```python
from build123d import *
from OCP.BRepFilletAPI import BRepFilletAPI_MakeChamfer

# Parameters (mm, degrees)
SKETCH1_R           = 0.85
BOSS_EXTRUDE1_DEPTH = 5
BOSS_EXTRUDE2_DEPTH = 2
SKETCH3_R           = 2.25
BOSS_EXTRUDE3_DEPTH = 5
SKETCH4_R           = 3.5
CUT_EXTRUDE1_DEPTH  = 3
SKETCH5_W           = 10
SKETCH5_H           = 10
CUT_EXTRUDE2_DEPTH  = 47.770717335
FILLET1_R           = 7
CHAMFER3_SIZE       = 0.5
CHAMFER1_SIZE       = 2.5
CHAMFER1_SIZE_2     = 1.25


with BuildPart() as part:
    # Sketch1 → Boss-Extrude1 (new body)
    with BuildSketch(Plane.XY):
        Polygon((-11, -35), (-11, 29), (10, 29), (10, -35), (17.5, -35), (17.5, 37.5), (-17.5, 37.5), (-17.5, -35), align=None)
        with Locations((-12.5, 32.5)):
            Circle(SKETCH1_R, mode=Mode.SUBTRACT)
        with Locations((12.5, 32.5)):
            Circle(SKETCH1_R, mode=Mode.SUBTRACT)
        with Locations((12.5, -32.5)):
            Circle(SKETCH1_R, mode=Mode.SUBTRACT)
    extrude(amount=BOSS_EXTRUDE1_DEPTH)

    # Sketch2 → Boss-Extrude2 (add)
    with BuildSketch(Plane.XY):
        Polygon((17.5, -35), (17.5, 37.5), (-17.5, 37.5), (-17.5, -35), (-15.1, -35), (-15.1, 35.1), (15.1, 35.1), (15.1, -35), align=None)
    extrude(amount=-BOSS_EXTRUDE2_DEPTH)

    # Sketch3 → Boss-Extrude3 (add)
    # profile 1 of 2: a face of its own
    with BuildSketch(Plane.XY):
        with BuildLine():
            Line((22.5, 5), (17.5, 5))
            Line((17.5, 5), (17.5, -5))
            Line((17.5, -5), (22.5, -5))
            ThreePointArc((22.5, -5), (27.5, 0), (22.5, 5))
        make_face()
        with Locations(Location((22.5, 0, 0), (0, 0, 180))):
            Circle(SKETCH3_R, mode=Mode.SUBTRACT)
    # profile 2 of 2: a face of its own
    with BuildSketch(Plane.XY):
        with BuildLine():
            Line((-22.5, 5), (-17.5, 5))
            Line((-17.5, 5), (-17.5, -5))
            Line((-17.5, -5), (-22.5, -5))
            ThreePointArc((-22.5, -5), (-27.5, 0), (-22.5, 5))
        make_face()
        with Locations(Location((-22.5, 0, 0), (0, 0, 180))):
            Circle(SKETCH3_R, mode=Mode.SUBTRACT)
    extrude(amount=BOSS_EXTRUDE3_DEPTH)

    # Sketch4 → Cut-Extrude1 (cut)
    with BuildSketch(Plane(origin=(0, 0, 0), x_dir=(-1, 0, 0), z_dir=(0, 0, -1))):
        with Locations((-22.5, 0)):
            Circle(SKETCH4_R)
        with Locations((22.5, 0)):
            Circle(SKETCH4_R)
    extrude(amount=-CUT_EXTRUDE1_DEPTH, mode=Mode.SUBTRACT)

    # Sketch5 → Cut-Extrude2 (cut, through all)
    with BuildSketch(Plane(origin=(0, 0, 0), x_dir=(-1, 0, 0), z_dir=(0, 0, -1))):
        with Locations((-12.5, 32.5)):
            Rectangle(SKETCH5_W, SKETCH5_H)
        with Locations((12.5, 32.5)):
            Rectangle(SKETCH5_W, SKETCH5_H)
    extrude(amount=CUT_EXTRUDE2_DEPTH, mode=Mode.SUBTRACT)

    # Fillet1
    fillet1_edges = [part.edges().sort_by_distance(p)[0] for p in [
        (-17.5, 37.5, 2.5),
        (17.5, 37.5, 2.5),
    ]]
    fillet(fillet1_edges, radius=FILLET1_R)

    # Chamfer3
    chamfer3_edges = [part.edges().sort_by_distance(p)[0] for p in [
        (-0.5, 29, 5),
        (-17.5, 17.75, 5),
        (0, 37.5, 5),
        (15.449747468, 35.449747468, 5),
        (-15.449747468, 35.449747468, 5),
        (10, -3, 5),
        (13.75, -35, 5),
        (-13.35, 32.5, 0),
        (-13.35, 32.5, 5),
        (17.5, -20, 5),
        (11.65, 32.5, 0),
        (11.65, 32.5, 5),
        (11.65, -32.5, 0),
        (11.65, -32.5, 5),
        (-14.25, -35, 5),
        (17.5, 17.75, 5),
        (27.5, 0, 5),
        (20, 5, 5),
        (20, -5, 5),
        (24.75, 0, 5),
        (-17.5, -20, 5),
        (-27.5, 0, 5),
        (-20, -5, 5),
        (-20, 5, 5),
        (-20.25, 0, 5),
        (-11, -3, 5),
    ]]
    chamfer(chamfer3_edges, length=CHAMFER3_SIZE)

    # Chamfer1
    chamfer1_edges_1 = [part.edges().sort_by_distance(p)[0] for p in [
        (26, 0, 3),
    ]]
    chamfer1_side_1 = [part.faces().sort_by_distance(p)[0] for p in [
        (26, 0, 2.975),
    ]]
    chamfer1_edges_2 = [part.edges().sort_by_distance(p)[0] for p in [
        (-19, 0, 3),
    ]]
    chamfer1_side_2 = [part.faces().sort_by_distance(p)[0] for p in [
        (-19, 0, 2.975),
    ]]
    chamfer1 = BRepFilletAPI_MakeChamfer(part.part.solid().wrapped)
    for e in chamfer1_edges_1:
        chamfer1.Add(CHAMFER1_SIZE - 0.0001, CHAMFER1_SIZE_2 - 0.0001, e.wrapped, chamfer1_side_1[0].wrapped)
    for e in chamfer1_edges_2:
        chamfer1.Add(CHAMFER1_SIZE - 0.0001, CHAMFER1_SIZE_2 - 0.0001, e.wrapped, chamfer1_side_2[0].wrapped)
    add(Compound.cast(chamfer1.Shape()), mode=Mode.REPLACE)  # a hair under: the kernel refuses the full size


solid = part.part
```
The listing builds one solid part. Answer for the finished solid, in the listing's coordinates (mm). A direction names the side the tool comes from. Round coordinates to 2 decimals unless told otherwise and drop trailing zeros. Order: outer loops, then holes, each group sorted by start corner. A loop starts at its lowest first (then second) coordinate and runs counter-clockwise, first axis right, second up. Notation, with made-up numbers: (-23, -39.75) -> (-15, -39.75) arc R15 ccw to (-15, -20.75) -> close; hole circle Ø1 at (40, 64.25). An arc over 180 degrees is marked (long way). Answer as CSV lines item,"result".
Q1. Which of the six approach directions +Z, -Z, +X, -X, +Y, -Y give full straight-line access (tool end or side, diameter ignored) to faces 4 (the flat face through (10, -3, 2)), 5 (the flat face through (20, -5, 2)), 6 (the flat face through (16, 27.5, -1)), 7 (the flat face through (0, 35.1, -1))?
Computed values:
face 4,"+Z, -Z, -Y"
face 5,"+Z, -Z, +X, -Y"
face 6,"-Z, +X, -X, +Y"
face 7,"-Z, +X, -X, -Y"
Q2. A cutting plane is placed at A-A on y = -29. Determine the outline of the cut face in (x, z), plus the area to 3 significant figures.
Computed values:
outline,"(-17.5, -2) -> (-15.1, -2) -> (-15.1, 0) -> (-11, 0) -> (-11, 4.5) -> (-11.5, 5) -> (-17, 5) -> (-17.5, 4.5) -> close; (10, 0) -> (15.1, 0) -> (15.1, -2) -> (17.5, -2) -> (17.5, 4.5) -> (17, 5) -> (10.5, 5) -> (10, 4.5) -> close"
area,"79.1 mm^2"
Q3. For a pull along X with two mould halves and no side action, classify faces 1 (the flat face through (20, 5, 2)), 2 (the conical face through (-15.14, 35.25, 4.86)), 3 (the flat face through (-1, 29, 2)) as +X half, -X half, draft (parallel to the pull), parting line (faces both ways), or undercut.
Computed values:
face 1,"draft"
face 2,"-X half"
face 3,"undercut"
Q4. A cutting plane is placed at B-B on z = -1.25. Determine the outline of the cut face in (x, y), plus the area to 3 significant figures.
Computed values:
outline,"(-17.5, -35) -> (-15.1, -35) -> (-15.1, 27.5) -> (-17.5, 27.5) -> close; (-7.5, 35.1) -> (7.5, 35.1) -> (7.5, 37.5) -> (-7.5, 37.5) -> close; (15.1, -35) -> (17.5, -35) -> (17.5, 27.5) -> (15.1, 27.5) -> close"
area,"336 mm^2"
Q5. A cutting plane is placed at C-C on x = 0. Determine the outline of the cut face in (y, z).
Computed values:
outline,"(29, 0) -> (35.1, 0) -> (35.1, -2) -> (37.5, -2) -> (37.5, 4.5) -> (37, 5) -> (29.5, 5) -> (29, 4.5) -> close"
Q6. Given pin 1 (1.6 mm diameter, centred on y = 35.5, z = -1, fed in from +X); pin 2 (0.6 mm diameter, centred on y = -12.5, z = -1, fed in from -X); pin 3 (1.3 mm diameter, centred on x = -21, z = 3, fed in from +Y), each flat-ended and moving along its own axis, determine where each tip first touches the part or whether it passes through.
Computed values:
pin 1,"stops at x = 7.5"
pin 2,"stops at x = -17.5"
pin 3,"stops at y = 5"
Q7. Consider line 1 (X direction, y = -32.5, z = 3.25); line 2 (X direction, y = 32.5, z = 1.85); line 3 (X direction, y = -3.5, z = -0.5). Determine where each line is inside the solid, lowest interval first. Write a range as from..to.
Computed values:
line 1,"x = -17.5..-11, 10..11.65, 13.35..17.5"
line 2,"x = -17.21..-13.35, -11.65..11.65, 13.35..17.21"
line 3,"x = -17.5..-15.1, 15.1..17.5"
Q8. A cutting plane is placed at D-D on y = 0. Give the number of separate pieces and of enclosed holes in the cut face, plus the area to 3 significant figures.
Computed values:
separate pieces,"4"
enclosed holes,"0"
area,"125 mm^2"
